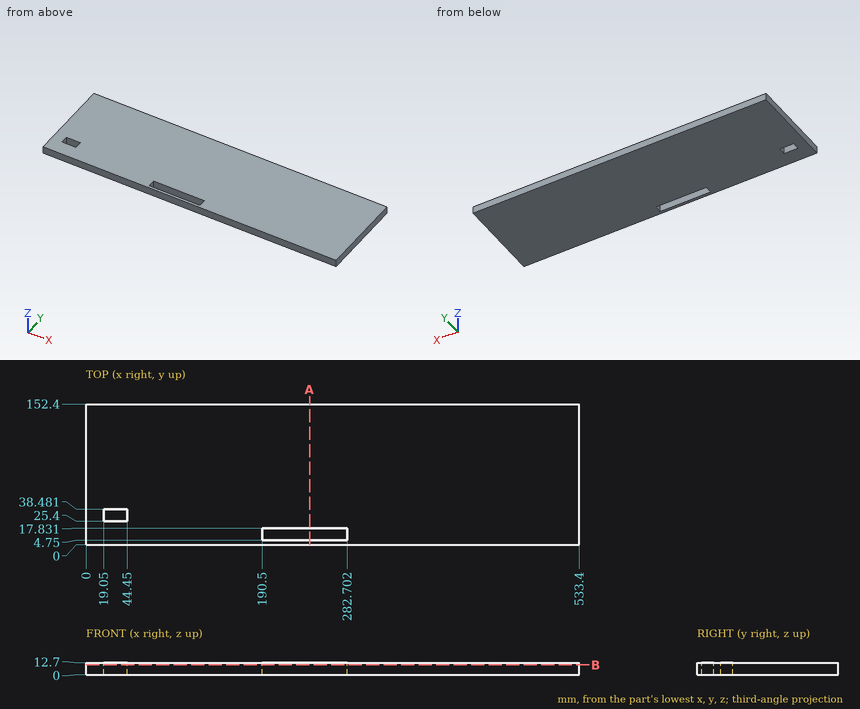
Verification items for this drawing (mm, ordinates from the low corner). Coordinates: 2 decimals unless noted, no trailing zeros. Write each loop counter-clockwise with the first axis right and the second up, starting at its lowest first coordinate (ties: lowest second). Pieces come first, ordered by that corner, then holes. Notation, with made-up numbers: M -25.5,-3.5 L 28.5,-3.5 A23 ccw 28.5,26.5 Z; hole C 62,87.25 d3. An arc over 180 degrees is marked long. One line per item, written item: value. Start each with the question number.
(1) Sectioned sample at B-B, the plane z = 10.5. Enter the section's corners in (x, y).
(2) Sectioned sample at A-A, the plane x = 242. Enter the section's corners in (y, z).
(3) Scan lines: line 1 along Y through (x, z) = (214, 7.5); line 2 along Y through (x, z) = (32, 9.5); line 3 along X through (y, z) = (37, 3.5). Record each from-to range of solid material in increasing order. Write a range as [from, to].
Filled sheet:
1. outline: M 0,0 L 533.4,0 L 533.4,152.4 L 0,152.4 Z; hole M 19.05,25.4 L 44.45,25.4 L 44.45,38.48 L 19.05,38.48 Z; hole M 190.5,4.75 L 282.7,4.75 L 282.7,17.83 L 190.5,17.83 Z
2. outline: M 0,0 L 4.75,0 L 4.75,12.7 L 0,12.7 Z; M 17.83,0 L 152.4,0 L 152.4,12.7 L 17.83,12.7 Z
3. line 1: [0, 4.75], [17.83, 152.4]
3. line 2: [0, 25.4], [38.48, 152.4]
3. line 3: [0, 19.05], [44.45, 533.4]
